```python
from build123d import *

# Parameters (mm, degrees)
AUFSATZ_LINEAR_AUSTRAGEN1_DEPTH = 3
SKIZZE2_W                       = 36
SKIZZE2_H                       = 1.5
SCHNITT_LINEAR_AUSTRAGEN1_DEPTH = 7


with BuildPart() as part:
    # Skizze1 → Aufsatz-Linear austragen1 (new body, symmetric)
    with BuildSketch(Plane.XY):
        with BuildLine():
            Line((-95, 7.6), (95, 7.6))
            ThreePointArc((95, 7.6), (102.6, 0), (95, -7.6))
            Line((95, -7.6), (-95, -7.6))
            ThreePointArc((-95, -7.6), (-102.6, 0), (-95, 7.6))
        make_face()
        with BuildLine():
            Line((-95, 6.1), (95, 6.1))
            ThreePointArc((95, 6.1), (101.1, 0), (95, -6.1))
            Line((95, -6.1), (-95, -6.1))
            ThreePointArc((-95, -6.1), (-101.1, 0), (-95, 6.1))
        make_face(mode=Mode.SUBTRACT)
    extrude(amount=AUFSATZ_LINEAR_AUSTRAGEN1_DEPTH, both=True)

    # Skizze2 → Schnitt-Linear austragen1 (cut, through all)
    with BuildSketch(Plane.XY.offset(3)):
        with Locations((0, 6.85)):
            Rectangle(SKIZZE2_W, SKIZZE2_H)
    extrude(amount=-SCHNITT_LINEAR_AUSTRAGEN1_DEPTH, mode=Mode.SUBTRACT)


solid = part.part
```
The model under review builds one solid part; all positions refer to its coordinate system, in mm. A direction names the side the tool comes from. Round coordinates to 2 decimals unless told otherwise and drop trailing zeros. Order: outer loops, then holes, each group sorted by start corner. A loop starts at its lowest first (then second) coordinate and runs counter-clockwise, first axis right, second up. Notation, with made-up numbers: (-14, -29.5) -> (14, -29.5) arc R14 ccw to (14, -21.5) -> close; hole circle Ø7 at (26.25, -4). An arc over 180 degrees is marked (long way). Use a Markdown table: item, result.
Q1. For line 1 (Y direction, x = 29.5, z = -0.35); line 2 (X direction, y = 0.5, z = 1.7); line 3 (X direction, y = 1.25, z = 1.5), list the stretches that pass through material, from the lowest coordinate up.
Values:
| item | result |
|---|---|
| line 1 | y = -7.6 to -6.1, 6.1 to 7.6 |
| line 2 | x = -102.58 to -101.08, 101.08 to 102.58 |
| line 3 | x = -102.5 to -100.97, 100.97 to 102.5 |
Q2. Tool access review of faces 1 (the flat face through (56, 6.1, 0)), 2 (the cylindrical face through (102.6, 0.17, 0.04)): name each direction out of +Z, -Z, +X, -X, +Y, -Y from which nothing blocks a thin tool from reaching the whole face with its end or side.
Values:
| item | result |
|---|---|
| face 1 | +Z, -Z |
| face 2 | +Z, -Z, +X |
Q3. We need section A-A on x = -40.5. Write out the cut boundary in (y, z).
Values:
| item | result |
|---|---|
| outline | (-7.6, -3) -> (-6.1, -3) -> (-6.1, 3) -> (-7.6, 3) -> close; (6.1, -3) -> (7.6, -3) -> (7.6, 3) -> (6.1, 3) -> close |
Q4. We need section B-B on y = 0. Write out the cut boundary in (x, z), then the cut area to 3 significant figures.
Values:
| item | result |
|---|---|
| outline | (-102.6, -3) -> (-101.1, -3) -> (-101.1, 3) -> (-102.6, 3) -> close; (101.1, -3) -> (102.6, -3) -> (102.6, 3) -> (101.1, 3) -> close |
| area | 18.0 mm^2 |
Q5. Clearance check with flat-ended pins moving along their axes: P1, Ø2, axis at y = -2, z = -2.5, coming from the +X side; P2, Ø1.6, axis at y = 6.5, z = 1.5, coming from the +X side. State where each tip first meets the part, or that it passes through.
Values:
| item | result |
|---|---|
| P1 | stops at x = 102.53 |
| P2 | stops at x = 100.03 |
Q6. We need section D-D on x = -11. Write out the cut boundary in (y, z), then the cut area to 3 significant figures.
Values:
| item | result |
|---|---|
| outline | (-7.6, -3) -> (-6.1, -3) -> (-6.1, 3) -> (-7.6, 3) -> close |
| area | 9.00 mm^2 |
Q7. We need section C-C on z = 1.95. Write out the cut boundary in (x, y).
Values:
| item | result |
|---|---|
| outline | (-95, -7.6) -> (95, -7.6) arc R7.6 ccw to (95, 7.6) -> (18, 7.6) -> (18, 6.1) -> (95, 6.1) arc R6.1 cw to (95, -6.1) -> (-95, -6.1) arc R6.1 cw to (-95, 6.1) -> (-18, 6.1) -> (-18, 7.6) -> (-95, 7.6) arc R7.6 ccw to start |
Q8. Mouldability with a two-part tool opening along Y and no side actions: class faces 3 (the flat face through (-57, 7.6, 0)), 4 (the cylindrical face through (-102.6, -0.17, 0.04)), 5 (the cylindrical face through (101.1, 0.1, 0)) as +Y half, -Y half, draft (parallel to the pull), parting line (faces both ways), or undercut.
Values:
| item | result |
|---|---|
| face 3 | +Y half |
| face 4 | parting line |
| face 5 | undercut |
